```python
from build123d import *

# Parameters (mm, degrees)
F0_W     = 40
F0_H     = 130
F1_DEPTH = 10
F2_R     = 5
F3_W     = 30
F3_H     = 20
F4_DEPTH = 25


with BuildPart() as f1:
    # F0 (on Top) → F1 (new body)
    with BuildSketch(Plane.XY):
        Rectangle(F0_W, F0_H)
    extrude(amount=F1_DEPTH)

    # F2
    f2_edges = [f1.edges().sort_by_distance(p)[0] for p in [
        (-20, -65, 5),
        (20, -65, 5),
        (20, 65, 5),
        (-20, 65, 5),
    ]]
    fillet(f2_edges, radius=F2_R)

    # F3 (on Top) → F4 (cut)
    with BuildSketch(Plane.XY):
        with Locations((0, 15)):
            Rectangle(F3_W, F3_H)
        with Locations((0, 45)):
            Rectangle(F3_W, F3_H)
        with Locations((0, -15)):
            Rectangle(F3_W, F3_H)
        with Locations((0, -45)):
            Rectangle(F3_W, F3_H)
    extrude(amount=F4_DEPTH, mode=Mode.SUBTRACT)


solid = f1.part
```
Can you work these out from the model? Positions are in its coordinate system, mm. A direction names the side the tool comes from. Give positions to 0.01 mm unless a question says otherwise; leave off trailing zeros. Write each loop counter-clockwise with the first axis right and the second up, starting at its lowest first coordinate (ties: lowest second). Pieces come first, ordered by that corner, then holes. Notation, with made-up numbers: (-11.5, 80) -> (6.5, 80) arc R24 ccw to (6.5, 101) -> close; hole circle Ø2 at (57.5, 70). An arc over 180 degrees is marked (long way). One line per item, written item: value.
Q1. Imagine slicing it at B-B on z = 7. Please give me the cut outline in (x, y).
Results found:
outline: (-20, -60) arc R5 ccw to (-15, -65) -> (15, -65) arc R5 ccw to (20, -60) -> (20, 60) arc R5 ccw to (15, 65) -> (-15, 65) arc R5 ccw to (-20, 60) -> close; hole (-15, -55) -> (15, -55) -> (15, -35) -> (-15, -35) -> close; hole (-15, -25) -> (15, -25) -> (15, -5) -> (-15, -5) -> close; hole (-15, 5) -> (15, 5) -> (15, 25) -> (-15, 25) -> close; hole (-15, 35) -> (15, 35) -> (15, 55) -> (-15, 55) -> close
Q2. Imagine slicing it at C-C on y = -39.5. Please give me the cut outline in (x, z).
Results found:
outline: (-20, 0) -> (-15, 0) -> (-15, 10) -> (-20, 10) -> close; (15, 0) -> (20, 0) -> (20, 10) -> (15, 10) -> close
Q3. Please list where these lines run through material, in increasing order: line 1 (Y direction, x = -11, z = 7.5); line 2 (X direction, y = 50.5, z = 8.75); line 3 (Y direction, x = 16.5, z = 6.75). Write a range as [from, to].
Results found:
line 1: y = [-65, -55], [-35, -25], [-5, 5], [25, 35], [55, 65]
line 2: x = [-20, -15], [15, 20]
line 3: y = [-64.77, 64.77]
Q4. Which directions (+Z, -Z, +X, -X, +Y, -Y) give clear straight access to the entire face, cutting with the end or side of a thin tool? Please do faces 1 (the face through (0, 1, 10)), 2 (the face through (0, 5, 5)).
Results found:
face 1: +Z, +X, -X, +Y, -Y
face 2: +Z, -Z
Q5. For P1, Ø10, axis at x = 16, y = -45, coming from the -Z side, with a flat end and sliding along its axis, tell me the tip position at first contact or that it passes through.
Results found:
P1: stops at z = 0
Q6. Imagine slicing it at A-A on x = 7. Please give me the cut outline in (y, z).
Results found:
outline: (-65, 0) -> (-55, 0) -> (-55, 10) -> (-65, 10) -> close; (-35, 0) -> (-25, 0) -> (-25, 10) -> (-35, 10) -> close; (-5, 0) -> (5, 0) -> (5, 10) -> (-5, 10) -> close; (25, 0) -> (35, 0) -> (35, 10) -> (25, 10) -> close; (55, 0) -> (65, 0) -> (65, 10) -> (55, 10) -> close
Q7. We'd pull the mould along Y, two halves only. Please class faces 3 (the face through (-19, -63, 5)), 4 (the face through (0, -25, 5)), 5 (the face through (0, 65, 5)): +Y half, -Y half, draft (parallel to the pull), parting line (faces both ways), or undercut.
Results found:
face 3: -Y half
face 4: undercut
face 5: +Y half
